Here's how the part is built. I have some questions about the finished solid (model axes, mm). Round coordinates to 2 decimals unless told otherwise and drop trailing zeros. Loops run counter-clockwise (first coordinate to the right, second up) from the corner with the lowest first, then second, coordinate; pieces in that order, holes last. Notation, with made-up numbers: (-33, 77.5) - (15, 77.5) arc R16 cw to (15, 104.5) - close; hole circle Ø1 at (-30, 89). An arc over 180 degrees is marked (long way). Return JSON: item names as keys, results as strings. Group by question number.
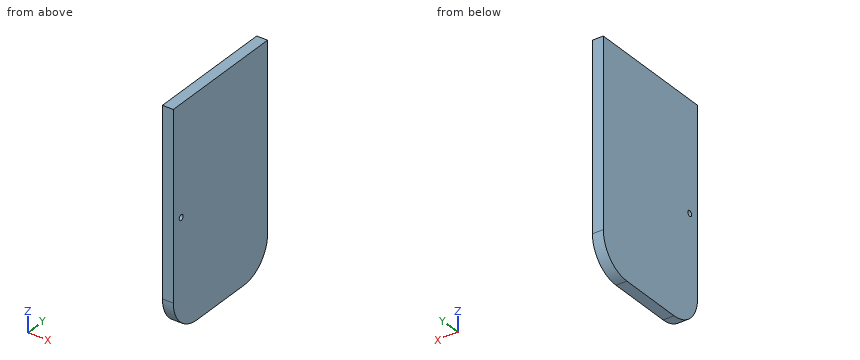
Autodesk Inventor part; units mm, degrees
ref_plane "YZ Plane" through (0, 0, 0) normal (1, 0, 0) x (0, 1, 0)
ref_plane "XZ Plane" through (0, 0, 0) normal (0, 1, 0) x (-1, 0, 0)
ref_plane "XY Plane" through (0, 0, 0) normal (0, 0, 1) x (1, 0, 0)
sketch "Sketch1" plane through (0, 0, 0) normal (1, 0, 0) x (0, 1, 0)
  line L0 (100.5124, 128.0095) -> (100.5124, -87.8905)
  line L1 (62.4124, -125.9905) -> (-13.7876, -125.9905)
  line L2 (-51.8876, -87.8905) -> (-51.8876, 128.0095)
  line L3 (-51.8876, 128.0095) -> (100.5124, 128.0095)
  arc A0 (62.4124, -125.9905) -> (100.5124, -87.8905) centre (62.4124, -87.8905) ccw
  arc A1 (-51.8876, -87.8905) -> (-13.7876, -125.9905) centre (-13.7876, -87.8905) ccw
  point P0 (0, 0)
  point P1 (100.5124, -125.9905)
  dimension "d0" = 254
  dimension "d1" = 152.4
  dimension "d3" = 38.1
extrude "Extrusion1" add sketch "Sketch1" along normal blind 12.7
sketch "Sketch3" plane through (12.7, 0, 0) normal (1, 0, 0) x (0, 0, -1)
  line L0 (125.9905, -13.7876) -> (125.9905, 62.4124)
  line L1 (-128.0095, 100.5124) -> (-128.0095, -51.8876)
  line L2 (-128.0095, -51.8876) -> (87.8905, -51.8876)
  point P0 (0, 0)
  point P1 (-1.0095, -39.1876)
  dimension "d16" = 254
  dimension "d17" = 127
  dimension "d18" = 12.7
hole "Hole2" at (12.7, -39.1876, 1.0095) direction (-1, 0, 0) diameter 6.35 end through all
Q1. Imagine slicing it at B-B, the plane y = 86.5. List the corners of the cut face in (x, z) for me, and give its area (3 significant figures).
Q2. Imagine slicing it at C-C, the plane y = -30.5. List the corners of the cut face in (x, z) for me, and give its area (3 significant figures).
Q3. Please list where these lines run through material, in increasing order: line 1 (Z direction, x = 4, y = 63.5); line 2 (Z direction, x = 11.5, y = 90.5).
Output values:
{
 "1": {"outline": "(0, -117.41) - (12.7, -117.41) - (12.7, 128.01) - (0, 128.01) - close", "area": "3,120 mm^2"},
 "2": {"outline": "(0, -122.13) - (12.7, -122.13) - (12.7, 128.01) - (0, 128.01) - close", "area": "3,180 mm^2"},
 "3": {"line 1": "z = -125.97 to 128.01", "line 2": "z = -113.63 to 128.01"}
}
